Answer from the drawing. Dimensions are ordinates in mm from the lowest x, y and z of the part. A direction names the side the tool comes from. Coordinates: 2 decimals unless noted, no trailing zeros. Order: outer loops, then holes, each group sorted by start corner. A loop starts at its lowest first (then second) coordinate and runs counter-clockwise, first axis right, second up. Notation, with made-up numbers: (-32.5, 72.5) -> (21.5, 72.5) arc R16 cw to (21.5, 101.5) -> close; hole circle Ø4 at (-8.5, 56.5). An arc over 180 degrees is marked (long way). Answer in a Markdown table with one row per item.
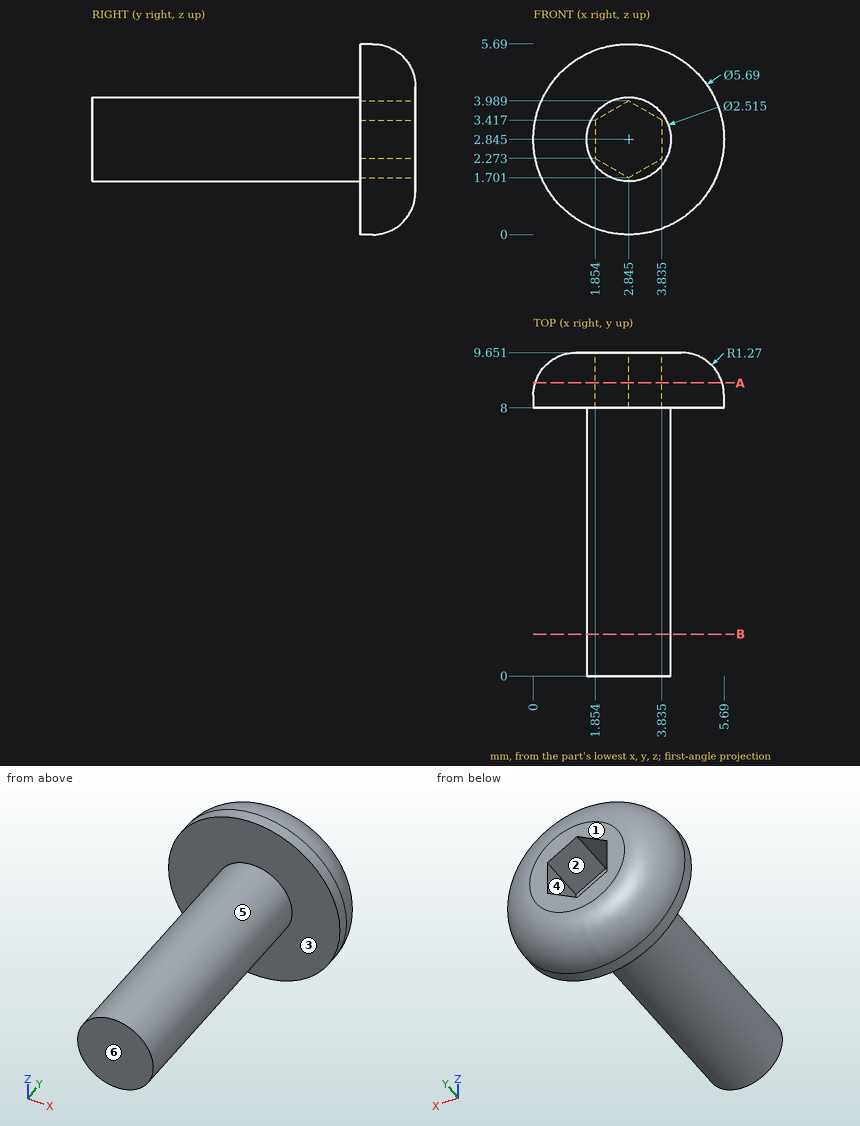
Q1. Given pin 1 (2 mm diameter, centred on y = 2.5, z = 3.5, fed in from -X); pin 2 (0.6 mm diameter, centred on x = 2.5, z = 3, fed in from +Y); pin 3 (0.6 mm diameter, centred on y = 8.5, z = 3, fed in from -X); pin 4 (1 mm diameter, centred on x = 2.5, y = 2.5, fed in from -Z), each flat-ended and moving along its own axis, determine where each tip first touches the part or whether it passes through.
Outcome:
| item | result |
|---|---|
| pin 1 | x = 1.59 |
| pin 2 | y = 8 |
| pin 3 | x = 0 |
| pin 4 | z = 1.59 |
Q2. Consider line 1 (X direction, y = 8.25, z = 3.15) (1 decimal); line 2 (Y direction, x = 1.45, z = 2.8); line 3 (X direction, y = 5, z = 2.9). Determine where each line is inside the solid, lowest interval first.
Outcome:
| item | result |
|---|---|
| line 1 | 0 to 1.9, 3.8 to 5.7 |
| line 2 | 8 to 9.65 |
| line 3 | 1.59 to 4.1 |
Q3. For the marked faces 1, 2 and 3, determine the directions among +Z, -Z, +X, -X, +Y, -Y from which every point of the face is accessible in a straight line to the end or side of a thin tool.
Outcome:
| item | result |
|---|---|
| face 1 | +Z, -Z, +X, -X, +Y |
| face 2 | +Y |
| face 3 | -Y |
Q4. For a pull along X with two mould halves and no side action, classify the marked faces 4, 5 and 6 as pulls with the +X half, pulls with the -X half, needs draft (parallel to the pull), parting line crosses it, or undercut.
Outcome:
| item | result |
|---|---|
| face 4 | undercut |
| face 5 | parting line crosses it |
| face 6 | needs draft |
Q5. The part is cut by section A-A (y = 8.75). Write down the section's boundary in (x, z) (1 decimal).
Outcome:
| item | result |
|---|---|
| outline | circle Ø5.6 at (2.8, 2.8); hole (1.9, 2.3) -> (2.8, 1.7) -> (3.8, 2.3) -> (3.8, 3.4) -> (2.8, 4) -> (1.9, 3.4) -> close |
Q6. The part is cut by section B-B (y = 1.25). Write down the section's boundary in (x, z) (1 decimal).
Outcome:
| item | result |
|---|---|
| outline | circle Ø2.5 at (2.8, 2.8) |
